CAD build for the part. Positions are in the model's coordinates, mm. A direction names the side the tool comes from. Give positions to 0.01 mm unless a question says otherwise; leave off trailing zeros. Order: outer loops, then holes, each group sorted by start corner. A loop starts at its lowest first (then second) coordinate and runs counter-clockwise, first axis right, second up.
```python
from build123d import *

# Parameters (mm, degrees)
F0_W     = 35.56
F0_H     = 35.56
F1_DEPTH = 5.08
F2_W     = 19.812
F2_H     = 4.572
F3_DEPTH = 2.54
F4_W     = 19.812
F4_H     = 4.572
F5_DEPTH = 2.54
F6_W     = 20.32
F6_H     = 5.08
F7_DEPTH = 2.54
F8_W     = 20.32
F8_H     = 5.08
F9_DEPTH = 2.54


with BuildPart() as f1:
    # F0 (on Top) → F1 (new body, symmetric)
    with BuildSketch(Plane.XY):
        Rectangle(F0_W, F0_H)
        with BuildLine():
            add(Edge.make_bspline(
                [(6.7551432292, 10.5116753472), (9.1391493056, 8.5383246528), (9.1391493056, 4.6302083333)],
                knots=[0, 0, 0, 1, 1, 1], degree=2))
            add(Edge.make_bspline(
                [(9.1391493056, 4.6302083333), (9.1391493056, 0.5622395833), (6.598046875, -1.5902560764)],
                knots=[0, 0, 0, 1, 1, 1], degree=2))
            add(Edge.make_bspline(
                [(6.598046875, -1.5902560764), (4.0569444444, -3.7427517361), (-0.6283854167, -3.7427517361)],
                knots=[0, 0, 0, 1, 1, 1], degree=2))
            Line((-0.6283854167, -3.7427517361), (-2.9159288194, -3.7427517361))
            Line((-2.9159288194, -3.7427517361), (-2.9159288194, -12.7))
            Line((-2.9159288194, -12.7), (-8.2572048611, -12.7))
            Line((-8.2572048611, -12.7), (-8.2572048611, 12.4850260417))
            Line((-8.2572048611, 12.4850260417), (-0.2149739583, 12.4850260417))
            add(Edge.make_bspline(
                [(-0.2149739583, 12.4850260417), (4.3711371528, 12.4850260417), (6.7551432292, 10.5116753472)],
                knots=[0, 0, 0, 1, 1, 1], degree=2))
        make_face(mode=Mode.SUBTRACT)
    extrude(amount=F1_DEPTH, both=True)

    # F2 (on face) → F3 (join)
    with BuildSketch(Plane(origin=(0, 17.78, 0), x_dir=(-1, 0, 0), z_dir=(0, 1, 0))):
        Rectangle(F2_W, F2_H)
    extrude(amount=F3_DEPTH)

    # F4 (on face) → F5 (join)
    with BuildSketch(Plane(origin=(-17.78, 0, 0), x_dir=(0, -1, 0), z_dir=(-1, 0, 0))):
        Rectangle(F4_W, F4_H)
    extrude(amount=F5_DEPTH)

    # F6 (on face) → F7 (cut)
    with BuildSketch(Plane.XZ.offset(17.78)):
        Rectangle(F6_W, F6_H)
    extrude(amount=-F7_DEPTH, mode=Mode.SUBTRACT)

    # F8 (on face) → F9 (cut)
    with BuildSketch(Plane.YZ.offset(17.78)):
        Rectangle(F8_W, F8_H)
    extrude(amount=-F9_DEPTH, mode=Mode.SUBTRACT)


solid = f1.part
```
Item 1: Wall check: L1, parallel to X at y = -5, z = 4.5; L2, parallel to X at y = 5, z = -0.25; L3, parallel to Y at x = -3.5, z = -4.25. Give the ranges that are in metal, low to high.
Item 2: Slice it at B-B (x = -1.5). Give the cut face in (y, z), and give its area (3 significant figures).
Item 3: Two-plate mould, pull along X, no slides. Class faces 1 (the face through (9.906, 19, 0)), 2 (the face through (0, 17.78, 3)), 3 (the face through (0, -17, -2.54)): released by +X, released by -X, zero draft, split by the parting line, or undercut.
Item 4: Slice it at A-A (y = -8.5). Give the cut face in (x, z).
Item 5: Slice it at C-C (x = -16). Give the cut face in (y, z).
Item 6: Drop flat-ended pins along their axis: pin 1 Ø3 at (x, y) = (-19, 0.5) entering from -Z; pin 2 Ø3 at (x, y) = (2.5, 19.5) entering from +Z; pin 3 Ø3 at (x, y) = (4.5, 19.5) entering from -Z; pin 4 Ø1.5 at (y, z) = (-0.5, -3.5) entering from -X. Give the stop position or say it passes through.
Item 7: Tool access for faces 4 (the face through (0, -17, 2.54)), 5 (the face through (-2, -3.743, 0)), 6 (the face through (-9.906, 19, 0)): list every direction of +Z, -Z, +X, -X, +Y, -Y with a clear straight run to the whole face (end or side of a thin tool).
A:
1. L1: x = -17.78 to -8.26, -2.92 to 17.78
1. L2: x = -20.32 to -8.26, 9.13 to 15.24
1. L3: y = -17.78 to -12.7, 12.49 to 17.78
2. outline: (-17.78, -5.08) - (-3.74, -5.08) - (-3.74, 5.08) - (-17.78, 5.08) - (-17.78, 2.54) - (-15.24, 2.54) - (-15.24, -2.54) - (-17.78, -2.54) - close; (12.49, -5.08) - (17.78, -5.08) - (17.78, -2.29) - (20.32, -2.29) - (20.32, 2.29) - (17.78, 2.29) - (17.78, 5.08) - (12.49, 5.08) - close
2. area: 195 mm2
3. face 1: released by +X
3. face 2: zero draft
3. face 3: undercut
4. outline: (-20.32, -2.29) - (-17.78, -2.29) - (-17.78, -5.08) - (-8.26, -5.08) - (-8.26, 5.08) - (-17.78, 5.08) - (-17.78, 2.29) - (-20.32, 2.29) - close; (-2.92, -5.08) - (17.78, -5.08) - (17.78, -2.54) - (15.24, -2.54) - (15.24, 2.54) - (17.78, 2.54) - (17.78, 5.08) - (-2.92, 5.08) - close
5. outline: (-17.78, -5.08) - (17.78, -5.08) - (17.78, 5.08) - (-17.78, 5.08) - close
6. pin 1: stops at z = -5.08
6. pin 2: stops at z = 2.29
6. pin 3: stops at z = -2.29
6. pin 4: stops at x = -17.78
7. face 4: -Y
7. face 5: +Z, -Z
7. face 6: +Z, -Z, -X, +Y
